Autodesk Inventor part; units mm, degrees
ref_plane "Work Plane1" through (-16.0653, -32.8267, -33.655) normal (0, 0, -1) x (0, 1, 0)
ref_plane "YZ Plane" through (0, 0, 0) normal (1, 0, 0) x (0, 1, 0)
ref_plane "XZ Plane" through (0, 0, 0) normal (0, 1, 0) x (-1, 0, 0)
sketch "Sketch1" plane through (0, 0, 0) normal (0, 0, 1) x (1, 0, 0)
  circle A0 centre (22.3624, 24.7247) radius 2.3813
  circle A1 centre (22.3624, -26.3473) radius 2.3813
  circle A2 centre (-9.3876, 24.7247) radius 2.3813
  circle A3 centre (-9.3876, -26.3473) radius 2.3813
  line L0 (28.7124, 32.6973) -> (-15.7376, 32.6973)
  line L1 (-15.7376, 32.6973) -> (-15.7376, -32.6973)
  line L2 (-15.7376, -32.6973) -> (28.7124, -32.6973)
  line L3 (28.7124, -32.6973) -> (28.7124, 32.6973)
  point P0 (0, 0)
extrude "Extrusion1" add sketch "Sketch1" along normal blind 12.7
sketch "Sketch2" plane through (-15.7376, -32.6973, 0) normal (0, -1, 0) x (1, 0, 0)
  line L0 (11.1075, 69.4178) -> (11.1075, 0)
  line L1 (33.3375, 69.1638) -> (33.3375, 0)
  line L2 (11.1075, 0) -> (33.3375, 0)
  line L3 (0, 9.525) -> (44.45, 9.525)
  line L4 (11.1075, 0) -> (33.3375, 0)
  line L5 (33.3375, 0) -> (33.3375, 5.334)
  line L6 (33.3375, 5.334) -> (11.1075, 5.334)
  line L7 (11.1075, 5.334) -> (11.1075, 0)
  line L8 (0, 0) -> (44.45, 0)
  point P0 (15.875, 0)
  point P1 (11.1075, 5.334)
  dimension "d2" = 5.334
  dimension "d21" = 0
extrude "Extrusion2" cut sketch "Sketch2" against normal blind 76.2 contours L6 L1 L2 L0
ref_plane "Work Plane1" through (-16.0653, -32.8267, -33.655) normal (0, 0, -1) x (0, 1, 0)
sketch "Sketch3" plane through (17.5999, -32.6973, 5.334) normal (0, 0, -1) x (-1, 0, 0)
  line L0 (0, 0) -> (0, 65.3946)
  line L1 (0, 46.9796) -> (22.23, 46.9796)
  line L2 (22.23, 46.9796) -> (22.23, 49.5196)
  line L3 (22.23, 49.5196) -> (0, 49.5196)
  line L4 (0, 49.5196) -> (0, 46.9796)
  line L5 (0, 65.3946) -> (22.23, 65.3946)
  line L6 (33.3375, 65.3946) -> (33.3375, 0)
  line L7 (0, 38.9796) -> (22.23, 38.9796)
  line L8 (22.23, 38.9796) -> (22.23, 41.5196)
  line L9 (22.23, 41.5196) -> (0, 41.5196)
  line L10 (0, 41.5196) -> (0, 38.9796)
  line L11 (0, 30.9796) -> (22.23, 30.9796)
  line L12 (22.23, 30.9796) -> (22.23, 33.5196)
  line L13 (22.23, 33.5196) -> (0, 33.5196)
  line L14 (0, 33.5196) -> (0, 30.9796)
  line L15 (0, 22.9796) -> (22.23, 22.9796)
  line L16 (22.23, 22.9796) -> (22.23, 25.5196)
  line L17 (22.23, 25.5196) -> (0, 25.5196)
  line L18 (0, 25.5196) -> (0, 22.9796)
  line L19 (0, 14.9796) -> (22.23, 14.9796)
  line L20 (22.23, 14.9796) -> (22.23, 17.5196)
  line L21 (22.23, 17.5196) -> (0, 17.5196)
  line L22 (0, 17.5196) -> (0, 14.9796)
  point P0 (17.5999, 32.6973)
  point P1 (0, 17.5196)
  point P2 (0, 14.9796)
  point P3 (0, 25.5196)
  point P4 (0, 22.9796)
  point P5 (0, 33.5196)
  point P6 (0, 30.9796)
  point P7 (0, 41.5196)
  point P8 (0, 38.9796)
  point P9 (0, 49.5196)
  dimension "d6" = 15.875
  dimension "d7" = 2.54
  dimension "d10" = 8
extrude "Extrusion3" add sketch "Sketch3" along normal blind 5.334
sketch "Sketch4" plane through (0, 0, 0) normal (0, 0, -1) x (-1, 0, 0)
  line L0 (4.6301, 14.2823) -> (4.6301, 16.8223)
  line L1 (15.7376, 32.6973) -> (15.7376, -32.6973)
  line L2 (4.6301, 16.8223) -> (15.7376, 16.8223)
  line L3 (15.7376, 16.8223) -> (15.7376, 19.9973)
  line L4 (15.7376, 19.9973) -> (4.6301, 19.9973)
  line L5 (4.6301, 19.9973) -> (4.6301, 16.8223)
  line L6 (4.6301, 14.2823) -> (4.6301, 8.8223)
  line L7 (4.6301, 6.2823) -> (4.6301, 0.8223)
  line L8 (4.6301, -1.7177) -> (4.6301, -7.1777)
  line L9 (4.6301, -9.7177) -> (4.6301, -15.1777)
  line L10 (-17.5999, 14.2823) -> (4.6301, 14.2823)
  line L11 (4.6301, 14.2823) -> (15.7376, 14.2823)
  line L12 (15.7376, 14.2823) -> (15.7376, 8.8223)
  line L13 (15.7376, 8.8223) -> (4.6301, 8.8223)
  line L14 (4.6301, 8.8223) -> (4.6301, 14.2823)
  line L15 (4.6301, 0.8223) -> (4.6301, 6.2823)
  line L16 (4.6301, 6.2823) -> (15.7376, 6.2823)
  line L17 (15.7376, 6.2823) -> (15.7376, 0.8223)
  line L18 (15.7376, 0.8223) -> (4.6301, 0.8223)
  line L19 (4.6301, 0.8223) -> (4.6301, 6.2823)
  line L20 (4.6301, -7.1777) -> (4.6301, -1.7177)
  line L21 (4.6301, -1.7177) -> (15.7376, -1.7177)
  line L22 (15.7376, -1.7177) -> (15.7376, -7.1777)
  line L23 (15.7376, -7.1777) -> (4.6301, -7.1777)
  line L24 (4.6301, -7.1777) -> (4.6301, -1.7177)
  line L25 (4.6301, -15.1777) -> (4.6301, -9.7177)
  line L26 (4.6301, -9.7177) -> (15.7376, -9.7177)
  line L27 (15.7376, -9.7177) -> (15.7376, -15.1777)
  line L28 (15.7376, -15.1777) -> (4.6301, -15.1777)
  line L29 (4.6301, -15.1777) -> (4.6301, -9.7177)
  line L30 (4.6301, -32.6973) -> (4.6301, -17.7177)
  line L31 (4.6301, -17.7177) -> (15.7376, -17.7177)
  line L32 (15.7376, -17.7177) -> (15.7376, -20.8927)
  line L33 (15.7376, -20.8927) -> (4.6301, -20.8927)
  line L34 (4.6301, -20.8927) -> (4.6301, -17.7177)
  line L35 (-28.7124, 32.6973) -> (15.7376, 32.6973) construction
  line L36 (-6.4874, 32.6973) -> (-6.4874, -33.4306) construction
  line L37 (-14.4, 16.8223) -> (-31.2231, 16.8223)
  line L38 (-31.2231, 16.8223) -> (-31.2231, 19.9973)
  line L39 (-31.2231, 19.9973) -> (-14.4, 19.9973)
  line L40 (-14.4, 19.9973) -> (-14.4, 16.8223)
  line L41 (-15.2764, -1.7177) -> (-15.2764, -7.1777)
  line L42 (-15.4955, -9.7177) -> (-15.4955, -15.1777)
  line L43 (-14.1435, 14.2823) -> (-30.6935, 14.2823)
  line L44 (-30.6935, 14.2823) -> (-30.6935, 8.8223)
  line L45 (-30.6935, 8.8223) -> (-16.0059, 8.8223)
  line L46 (-16.0059, 8.8223) -> (-14.1435, 14.2823)
  line L47 (-10.7606, 6.2823) -> (-30.4287, 6.2823)
  line L48 (-30.4287, 6.2823) -> (-30.4287, 0.8223)
  line L49 (-30.4287, 0.8223) -> (-15.6598, 0.8223)
  line L50 (-15.6598, 0.8223) -> (-10.7606, 6.2823)
  line L51 (-15.2764, -7.1777) -> (-15.2764, -1.7177)
  line L52 (-15.2764, -1.7177) -> (-29.0132, -1.7177)
  line L53 (-29.0132, -1.7177) -> (-29.0132, -7.1777)
  line L54 (-29.0132, -7.1777) -> (-15.2764, -7.1777)
  line L55 (-15.2764, -7.1777) -> (-15.2764, -1.7177)
  line L56 (-15.4955, -15.1777) -> (-15.4955, -9.7177)
  line L57 (-15.4955, -9.7177) -> (-29.8897, -9.7177)
  line L58 (-29.8897, -9.7177) -> (-29.8897, -15.1777)
  line L59 (-29.8897, -15.1777) -> (-15.4955, -15.1777)
  line L60 (-15.4955, -15.1777) -> (-15.4955, -9.7177)
  line L61 (-15.5503, -17.7177) -> (-32.0838, -17.7177)
  line L62 (-32.0838, -17.7177) -> (-32.0838, -20.8927)
  line L63 (-32.0838, -20.8927) -> (-15.5503, -20.8927)
  line L64 (-15.5503, -20.8927) -> (-15.5503, -17.7177)
  point P0 (0, 0)
  point P1 (-15.4955, -15.1777)
  point P2 (-15.2764, -7.1777)
  point P3 (4.6301, -20.8927)
  point P4 (15.7376, -17.7177)
  point P5 (4.6301, -15.1777)
  point P6 (15.7376, -9.7177)
  point P7 (15.7376, -1.7177)
  point P8 (4.6301, 0.8223)
  point P9 (15.7376, 6.2823)
  point P10 (4.6301, 8.8223)
  point P11 (15.7376, 14.2823)
  point P12 (15.7376, 16.8223)
  dimension "d17" = 3.175
  dimension "d18" = 3.175
extrude "Extrusion4" cut sketch "Sketch4" against normal blind 5.334 contours L1 L33 L30 L31 | L1 L28 L9 L26 | L1 L23 L8 L21 | L1 L18 L7 L16 | L11 L1 L13 L6 | L46 L45 L44 L43 L10 | L5 L4 L1 L2 | L37 L38 L39 L40 | L41 L54 L53 L52 | L42 L59 L58 L57 | L50 L49 L48 L47 | L64 L63 L62 L61
sketch "Sketch5" plane through (0, 0, 0) normal (0, 0, -1) x (-1, 0, 0)
  line L0 (17.6982, 19.0646) -> (-30.6897, 19.0646)
  line L1 (-30.6897, 19.0646) -> (-30.6897, -19.7169)
  line L2 (-30.6897, -19.7169) -> (17.6982, -19.7169)
  line L3 (17.6982, -19.7169) -> (17.6982, 19.0646)
extrude "Extrusion5" cut sketch "Sketch5" against normal blind 2.159
properties part number "Belt Clamp"
Model file for the job. Use its own axes, mm. A direction names the side the tool comes from. Give positions to 0.01 mm unless a question says otherwise; leave off trailing zeros. Write each loop counter-clockwise with the first axis right and the second up, starting at its lowest first coordinate (ties: lowest second). Pieces come first, ordered by that corner, then holes. Notation, with made-up numbers: M 25.5,-13 L 29.5,-13 A30 cw 29.5,20 Z; hole C 66,-18 d3. An arc over 180 degrees is marked long. One line per item, written item: value. Start each with the question number.
Q1. Saw through at D-D, the plane z = 8.5. Write the cut outline in (x, y), plus the area to 3 significant figures.
Q2. 3-axis set-ups, long thin cutter, end or side, ignore diameter. For faces 4 (the flat face through (-11.5, -28, 0)), 5 (the flat face through (7, -12, 5.334)): which of +Z, -Z, +X, -X, +Y, -Y reach the whole face in a straight line?
Q3. Saw through at B-B, the plane x = 0.5. Write the cut outline in (y, z).
Q4. Probe probe 1 along Y at (x, z) = (17, 2.75); probe 2 along X at (y, z) = (25, 8.75); probe 3 along Y at (x, z) = (-8, 11.5). List the from-to ranges inside material, lowest first. Write a range as [from, to].
Q5. Saw through at C-C, the plane y = 23. Write the cut outline in (x, z), plus the area to 3 significant figures.
Q6. Drop flat-ended pins along their axis: pin 1 Ø6 at (x, y) = (10.5, -4.5) entering from -Z; pin 2 Ø3.5 at (x, z) = (10.5, 3) entering from +Y; pin 3 Ø2.5 at (x, y) = (11.5, 12.5) entering from -Z. Give the stop position or say it passes through.
Q7. Two-plate mould, pull along X, no slides. Class faces 1 (the flat face through (24.3, -28, 0)), 2 (the flat face through (-15.738, 0, 8)), 3 (the cylindrical face through (-11.143, 23.115, 6.261)): +X half, -X half, draft (parallel to the pull), parting line (faces both ways), or undercut.
Q8. Saw through at A-A, the plane z = 1. Write the cut outline in (x, y), plus the area to 3 significant figures.
Output values:
1. outline: M -15.74,-32.7 L 28.71,-32.7 L 28.71,32.7 L -15.74,32.7 Z; hole C -9.39,-26.35 d4.76; hole C -9.39,24.72 d4.76; hole C 22.36,-26.35 d4.76; hole C 22.36,24.72 d4.76
1. area: 2,840 mm²
2. face 4: -Z, +X, -X, +Y, -Y
2. face 5: -Z, +X, -X
3. outline: M -32.7,5.33 L -17.72,5.33 L -17.72,2.16 L -15.18,2.16 L -15.18,5.33 L -9.72,5.33 L -9.72,2.16 L -7.18,2.16 L -7.18,5.33 L -1.72,5.33 L -1.72,2.16 L 0.82,2.16 L 0.82,5.33 L 6.28,5.33 L 6.28,2.16 L 8.82,2.16 L 8.82,5.33 L 14.28,5.33 L 14.28,2.16 L 16.82,2.16 L 16.82,5.33 L 32.7,5.33 L 32.7,12.7 L -32.7,12.7 Z
4. probe 1: y = [-17.72, -15.18], [-9.72, -7.18], [-1.72, 0.82], [6.28, 8.82], [14.28, 16.82]
4. probe 2: x = [-15.74, -11.75], [-7.02, 20], [24.73, 28.71]
4. probe 3: y = [-32.7, -28.28], [-24.41, 22.79], [26.66, 32.7]
5. outline: M -15.74,0 L -11.03,0 L -11.03,12.7 L -15.74,12.7 Z; M -7.75,0 L -4.63,0 L -4.63,5.33 L 17.6,5.33 L 17.6,0 L 20.72,0 L 20.72,12.7 L -7.75,12.7 Z; M 24,0 L 28.71,0 L 28.71,12.7 L 24,12.7 Z
5. area: 363 mm²
6. pin 1: stops at z = 2.16
6. pin 2: stops at y = 16.82
6. pin 3: stops at z = 5.33
7. face 1: draft
7. face 2: -X half
7. face 3: undercut
8. outline: M -15.74,-32.7 L -4.63,-32.7 L -4.63,-20.89 L -15.74,-20.89 Z; M -15.74,20 L -4.63,20 L -4.63,32.7 L -15.74,32.7 Z; M 17.6,-32.7 L 28.71,-32.7 L 28.71,-20.89 L 17.6,-20.89 Z; M 17.6,20 L 28.71,20 L 28.71,32.7 L 17.6,32.7 Z; hole C -9.39,-26.35 d4.76; hole C -9.39,24.72 d4.76; hole C 22.36,-26.35 d4.76; hole C 22.36,24.72 d4.76
8. area: 473 mm²
